Design review of the part built by this model. Coordinates are the model's own, in mm. A direction names the side the tool comes from. Give positions to 0.01 mm unless a question says otherwise; leave off trailing zeros. Write each loop counter-clockwise with the first axis right and the second up, starting at its lowest first coordinate (ties: lowest second). Pieces come first, ordered by that corner, then holes. Notation, with made-up numbers: M 57,-10.5 L 94,-10.5 A16 cw 94,-6.5 Z; hole C -35.75,-27.5 d10. An arc over 180 degrees is marked long. Use one line per item in the form item = value. Start each with the question number.
from build123d import *

# Parameters (mm, degrees)
SKETCH1_R           = 6.223
SKETCH1_R_2         = 4.7625
BOSS_EXTRUDE1_DEPTH = 52.959
SKETCH2_R           = 6.35
SKETCH2_R_2         = 5.9436
CUT_EXTRUDE1_DEPTH  = 0.9906


with BuildPart() as part:
    # Sketch1 → Boss-Extrude1 (new body, symmetric)
    with BuildSketch(Plane(origin=(0, 0, 0), x_dir=(0, 0, -1), z_dir=(1, 0, 0))):
        Circle(SKETCH1_R)
        Circle(SKETCH1_R_2, mode=Mode.SUBTRACT)
    extrude(amount=BOSS_EXTRUDE1_DEPTH, both=True)

    # Sketch2 → Cut-Extrude1 (cut)
    with BuildSketch(Plane.ZY.offset(51.054)):
        Circle(SKETCH2_R)
        Circle(SKETCH2_R_2, mode=Mode.SUBTRACT)
    cut_extrude1 = extrude(amount=CUT_EXTRUDE1_DEPTH, mode=Mode.SUBTRACT)

    # Mirror1: Cut-Extrude1 across plane
    add(cut_extrude1.mirror(Plane(origin=(0, 0, 0), x_dir=(0, 0, 1), z_dir=(1, 0, 0))), mode=Mode.SUBTRACT)


solid = part.part
1. Draft analysis for pull direction X (two halves, no side actions). For faces 3 (the flat face through (52.959, -5, 1)), 4 (the cylindrical face through (51.542, 1.785, 5.669)), 5 (the cylindrical face through (0.715, -6.075, 1.349)), state which applies: pulls with the +X half, pulls with the -X half, needs draft (parallel to the pull), parting line crosses it, or undercut.
2. For faces 1 (the cylindrical face through (-51.542, 1.785, 5.669)), 2 (the cylindrical face through (52.508, -6.075, 1.349)), list the 3-axis set-ups (+Z, -Z, +X, -X, +Y, -Y) from which the entire face can be reached by the end or side of a thin tool; tool diameter is ignored.
3. We need section A-A (z = 0). State the section outline as (x, y) points, and give its area (3 significant figures).
4. Clearance check with flat-ended pins moving along their axes: pin 1 Ø3 at (x, z) = (-25.5, -4.5) entering from -Y; pin 2 Ø3 at (x, z) = (12, 2) entering from -Y; pin 3 Ø4 at (x, y) = (-28, 4) entering from +Z. State where each tip first meets the part, or that it passes through.
5. We need section C-C (x = 8). State the section outline as (y, z) points (1 decimal).
6. To check wall thickness, follow L1, parallel to Y at x = 5, z = 0; L2, parallel to Z at x = -40.5, y = -3.5; L3, parallel to Z at x = 37.5, y = 2.25. State the ranges of each line that lie inside material, in increasing order.
Answer block:
q1.face_3 = pulls with the +X half
q1.face_4 = undercut
q1.face_5 = needs draft
q2.face_1 = none
q2.face_2 = +X, -X
q3.outline = M -52.96,-6.22 L -52.04,-6.22 L -52.04,-5.94 L -51.05,-5.94 L -51.05,-6.22 L 51.05,-6.22 L 51.05,-5.94 L 52.04,-5.94 L 52.04,-6.22 L 52.96,-6.22 L 52.96,-4.76 L -52.96,-4.76 Z; M -52.96,4.76 L 52.96,4.76 L 52.96,6.22 L 52.04,6.22 L 52.04,5.94 L 51.05,5.94 L 51.05,6.22 L -51.05,6.22 L -51.05,5.94 L -52.04,5.94 L -52.04,6.22 L -52.96,6.22 Z
q3.area = 308 mm^2
q4.pin_1 = -5.45
q4.pin_2 = -6.2
q4.pin_3 = 5.89
q5.outline = C 0,0 d12.4; hole C 0,0 d9.5
q6.L1 = -6.22 to -4.76, 4.76 to 6.22
q6.L2 = -5.15 to -3.23, 3.23 to 5.15
q6.L3 = -5.8 to -4.2, 4.2 to 5.8
